Autodesk Inventor part; units mm, degrees
ref_plane "YZ Plane" through (0, 0, 0) normal (1, 0, 0) x (0, 1, 0)
ref_plane "XZ Plane" through (0, 0, 0) normal (0, 1, 0) x (-1, 0, 0)
ref_plane "XY Plane" through (0, 0, 0) normal (0, 0, 1) x (1, 0, 0)
sketch "Sketch3" plane through (0, 0, 0) normal (0, 0, 1) x (1, 0, 0)
  circle A0 centre (0, 0) radius 8
  dimension "d1" = 16
extrude "Extrusion1" add sketch "Sketch3" against normal blind 11.75
sketch "Sketch4" plane through (0, 0, -11.75) normal (0, 0, -1) x (-1, 0, 0)
  line L0 (-5.4028, 5.9) -> (5.4028, 5.9)
  circle A0 centre (0, 0) radius 8
  line L1 (-5.4028, -5.9) -> (5.4028, -5.9)
  line L2 (0, 5.9) -> (0, -5.9)
  dimension "d6" = 11.8
extrude "Extrusion2" add sketch "Sketch4" along normal blind 26.5 contours L0 L2 L1 A0 | L0 A0 L1 L2
sketch "Sketch5" plane through (0, 0, 0) normal (0, 0, 1) x (1, 0, 0)
  circle A0 centre (0, 0) radius 3
  dimension "d9" = 6
extrude "Extrusion3" add sketch "Sketch5" along normal blind 2
sketch "Sketch6" plane through (0, 0, 2) normal (0, 0, 1) x (1, 0, 0)
  circle A0 centre (0, 0) radius 1.5
  line L0 (0, -11.2) -> (0, 11.2)
  line L1 (1, 1.118) -> (1, -1.118)
  dimension "d12" = 3
  dimension "d13" = 1
extrude "Extrusion4" add sketch "Sketch6" along normal blind 8 contours L1 A0 L0 | L0 A0
sketch "Sketch7" plane through (0, 0, -38.25) normal (0, 0, -1) x (-1, 0, 0)
  circle A0 centre (0, 0) radius 2.95
  dimension "d16" = 5.9
extrude "Extrusion5" add sketch "Sketch7" along normal blind 1.5
sketch "Sketch10" plane through (0, 0, -38.25) normal (0, 0, -1) x (-1, 0, 0)
  line L0 (-6.5, -1) -> (-6.25, -1)
  line L1 (-6.25, -1) -> (-6.25, 1)
  line L2 (-6.25, 1) -> (-6.5, 1)
  line L3 (-6.5, 1) -> (-6.5, -1)
  line L4 (-6.5, -1) -> (-6.25, 1) construction
  line L5 (-6.25, -1) -> (-6.5, 1) construction
  line L6 (11.2, 0) -> (-11.2, 0)
  line L7 (0, -11.2) -> (0, 11.2)
  line L8 (6.5, -1) -> (6.25, -1)
  line L9 (6.25, -1) -> (6.25, 1)
  line L10 (6.25, 1) -> (6.5, 1)
  line L11 (6.5, 1) -> (6.5, -1)
  point P0 (0, 0)
  point P1 (-6.375, 0)
  point P2 (-6.375, 0)
  dimension "d23" = 0.25
  dimension "d24" = 2
  dimension "d25" = 13
extrude "Extrusion7" add sketch "Sketch10" along normal blind 3.5
fillet "Fillet2" radius 0.8 4 edges at (-6.375, 1, -41.75) (-6.375, -1, -41.75) (6.375, 1, -41.75) (6.375, -1, -41.75)
properties part number "DriveMotorV1" material "Motor"
CAD build for the part. Positions are in the model's coordinates, mm. A direction names the side the tool comes from. Round coordinates to 2 decimals unless told otherwise and drop trailing zeros. Order: outer loops, then holes, each group sorted by start corner. A loop starts at its lowest first (then second) coordinate and runs counter-clockwise, first axis right, second up. Notation, with made-up numbers: (14, 41) -> (65, 41) arc R16 cw to (65, 52) -> close; hole circle Ø6 at (-6, 13.5). An arc over 180 degrees is marked (long way). Write item = value, one per line. Start each with the question number.
(1) Cut at D-D, the plane x = 4.25. List the corners of the cut face in (y, z), then the cut area to 3 significant figures.
(2) Pull direction X, two halves, no side cores. Call faces 1 (the flat face through (0, 0, -39.75)), 2 (the flat face through (6.25, 0, -40)), 3 (the flat face through (-6.5, 0, -40)), 4 (the flat face through (6.5, 0, -40)): released by +X, released by -X, zero draft, split by the parting line, or undercut.
(3) Cut at B-B, the plane y = -2. List the corners of the cut face in (x, z), then the cut area to 3 significant figures.
(4) Cut at A-A, the plane x = 0. List the corners of the cut face in (y, z), then the cut area to 3 significant figures.
(5) Pin check, flat tips, straight feed: P1, Ø3.5, axis at x = 4, y = 2, coming from the -Z side; P2, Ø1.5, axis at x = 4.5, z = 4, coming from the -Y side; P3, Ø1.1, axis at x = 1, y = -6.5, coming from the -Z side; P4, Ø1, axis at y = -0.5, z = -39, coming from the +X side. Stop position of each tip, or through.
(6) Probe line 1 (Z direction, x = 4, y = 1.25); line 2 (Z direction, x = 1.5, y = 6.5); line 3 (Y direction, x = 4.25, z = -17). List the from-to ranges inside material, lowest first. Write a range as [from, to].
(7) Cut at C-C, the plane z = -7.5. List the corners of the cut face in (x, y), then the cut area to 3 significant figures.
(8) Which spindle directions (+Z, -Z, +X, -X, +Y, -Y) get a long thin tool onto all of the face, cutting with end or side? Do faces 5 (the cylindrical face through (2.947, -0.13, -38.99)), 6 (the flat face through (3.4, 0.1, 0)), 7 (the flat face through (-6.25, 0, -40)). Say none if no direction does.
Model answer:
q1.outline = (-6.78, -11.75) -> (-5.9, -11.75) -> (-5.9, -38.25) -> (5.9, -38.25) -> (5.9, -11.75) -> (6.78, -11.75) -> (6.78, 0) -> (-6.78, 0) -> close
q1.area = 472 mm2
q2.face_1 = undercut
q2.face_2 = undercut
q2.face_3 = released by -X
q2.face_4 = released by +X
q3.outline = (-7.75, -38.25) -> (-2.17, -38.25) -> (-2.17, -39.75) -> (2.17, -39.75) -> (2.17, -38.25) -> (7.75, -38.25) -> (7.75, 0) -> (2.24, 0) -> (2.24, 2) -> (-2.24, 2) -> (-2.24, 0) -> (-7.75, 0) -> close
q3.area = 608 mm2
q4.outline = (-8, -11.75) -> (-5.9, -11.75) -> (-5.9, -38.25) -> (-2.95, -38.25) -> (-2.95, -39.75) -> (2.95, -39.75) -> (2.95, -38.25) -> (5.9, -38.25) -> (5.9, -11.75) -> (8, -11.75) -> (8, 0) -> (3, 0) -> (3, 2) -> (1.5, 2) -> (1.5, 10) -> (-1.5, 10) -> (-1.5, 2) -> (-3, 2) -> (-3, 0) -> (-8, 0) -> close
q4.area = 546 mm2
q5.P1 = -39.75
q5.P2 = through
q5.P3 = -11.75
q5.P4 = 6.5
q6.line_1 = [-38.25, 0]
q6.line_2 = [-11.75, 0]
q6.line_3 = [-5.9, 5.9]
q7.outline = circle Ø16 at (0, 0)
q7.area = 201 mm2
q8.face_5 = -Z
q8.face_6 = +Z
q8.face_7 = -Z, +Y, -Y
